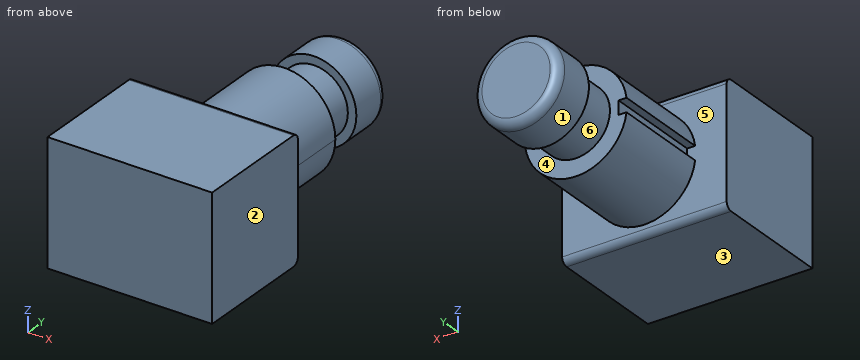
Autodesk Inventor part; units mm, degrees
ref_plane "YZ Plane" through (0, 0, 0) normal (1, 0, 0) x (0, 1, 0)
ref_plane "XZ Plane" through (0, 0, 0) normal (0, 1, 0) x (-1, 0, 0)
ref_plane "XY Plane" through (0, 0, 0) normal (0, 0, 1) x (1, 0, 0)
sketch "Sketch1" plane through (0, 0, 0) normal (0, 1, 0) x (-1, 0, 0)
  line L0 (9.65, 7.25) -> (-9.65, 7.25)
  line L1 (-9.65, 7.25) -> (-9.65, -7.25)
  line L2 (-9.65, -7.25) -> (9.65, -7.25)
  line L3 (9.65, -7.25) -> (9.65, 7.25)
  line L4 (9.65, 7.25) -> (-9.65, -7.25) construction
  line L5 (-9.65, 7.25) -> (9.65, -7.25) construction
  point P0 (0, 0)
  dimension "d0" = 19.3
  dimension "d1" = 14.5
extrude "Extrusion1" add sketch "Sketch1" along normal blind 14.5
sketch "Sketch2" plane through (0, 14.5, 0) normal (0, 1, 0) x (1, 0, 0)
  circle A0 centre (0, 0) radius 6
  line L0 (-6.9823, -0.8) -> (-5.0177, -0.8)
  line L1 (-5.0177, -0.8) -> (-5.0177, 0.8)
  line L2 (-5.0177, 0.8) -> (-6.9823, 0.8)
  line L3 (-6.9823, 0.8) -> (-6.9823, -0.8)
  line L4 (-6.9823, -0.8) -> (-5.0177, 0.8) construction
  line L5 (-5.0177, -0.8) -> (-6.9823, 0.8) construction
  point P0 (-6, 0)
  point P1 (5.9823, -0.4609)
  point P2 (-5.9464, -0.8)
  point P3 (-5.9464, 0.8)
  dimension "d4" = 12
  dimension "d5" = 1.6
  dimension "d6" = 11
extrude "Extrusion2" add sketch "Sketch2" along normal blind 11.6 contours A0 L0 L1 L2 picked at (-1.3451, 0)
sketch "Sketch3" plane through (0, 26.1, 0) normal (0, 1, 0) x (1, 0, 0)
  circle A0 centre (0, 0) radius 4
  dimension "d9" = 8
extrude "Extrusion3" add sketch "Sketch3" along normal blind 5
sketch "Sketch4" plane through (0, 31.1, 0) normal (0, 1, 0) x (1, 0, 0)
  circle A0 centre (0, 0) radius 5
  dimension "d12" = 10
extrude "Extrusion4" add sketch "Sketch4" along normal blind 5.1
fillet "Fillet1" radius 1 1 edges at (-5, 36.2, 0)
thread "Thread1"
fillet "Fillet2" radius 0.75 2 edges at (0, 14.5, 7.25) (0, 14.5, -7.25)
properties part number "ar70736"
The listing builds one solid part. Answer for the finished solid, in the listing's coordinates (mm). Face numbers are marked on the shaded views. A direction names the side the tool comes from. Coordinates: 2 decimals unless noted, no trailing zeros. Loops run counter-clockwise (first coordinate to the right, second up) from the corner with the lowest first, then second, coordinate; pieces in that order, holes last. Notation, with made-up numbers: (76, 80) -> (122, 80) arc R20 ccw to (122, 112) -> close; hole circle Ø9 at (58.5, 14.5). An arc over 180 degrees is marked (long way). Use one line per item in the form item = value. Start each with the question number.
Item 1: The part is cut by section C-C on y = 19.5. Determine the outline of the cut face in (x, z).
Item 2: The part is cut by section D-D on x = 0. Determine the outline of the cut face in (y, z).
Item 3: A tool of negligible diameter and unlimited length cuts with its end or side. For the marked faces 1 and 2, from which of +Z, -Z, +X, -X, +Y, -Y can it reach the whole face along a straight path? Write none if from no direction.
Item 4: Flat-ended cylindrical pins translate along their axes: pin 1 Ø0.5 at (x, y) = (-5.5, 18) entering from -Z; pin 2 Ø3 at (x, y) = (0.5, 29) entering from +Z; pin 3 Ø3 at (x, z) = (-6.5, 2) entering from +Y. Find the tip coordinate at first contact, or state that the pin passes through.
Item 5: The mould has two halves that part along Y. Classify the marked faces 3, 4, 5 and 6: released by +Y, released by -Y, zero draft, split by the parting line, or undercut.
Item 6: Consider L1, parallel to Y at x = 5.5, z = 6.25; L2, parallel to Y at x = 3.5, z = -4; L3, parallel to Z at x = 4, y = 24. Determine where each line is inside the solid, lowest interval first. Write a range as [from, to].
Item 7: The part is cut by section A-A on x = 7.5. Determine the outline of the cut face in (y, z), then the cut area to 3 significant figures.
Item 8: The part is cut by section B-B on z = 5.5. Determine the outline of the cut face in (x, y), then the cut area to 3 significant figures.
Answer key:
q1.outline = (-5.95, -0.8) arc R6 ccw (long way) to (-5.95, 0.8) -> (-5.02, 0.8) -> (-5.02, -0.8) -> close
q2.outline = (0, -7.25) -> (13.75, -7.25) arc R0.75 ccw to (14.5, -6.5) -> (14.5, -6) -> (26.1, -6) -> (26.1, -4) -> (31.1, -4) -> (31.1, -5) -> (35.2, -5) arc R1 ccw to (36.2, -4) -> (36.2, 4) arc R1 ccw to (35.2, 5) -> (31.1, 5) -> (31.1, 4) -> (26.1, 4) -> (26.1, 6) -> (14.5, 6) -> (14.5, 6.5) arc R0.75 ccw to (13.75, 7.25) -> (0, 7.25) -> close
q3.face_1 = +Y
q3.face_2 = +Z, -Z, +X, +Y, -Y
q4.pin_1 = -2.9
q4.pin_2 = 4
q4.pin_3 = 26.1
q5.face_3 = zero draft
q5.face_4 = undercut
q5.face_5 = released by +Y
q5.face_6 = undercut
q6.L1 = [0, 14.5]
q6.L2 = [0, 26.1]
q6.L3 = [-4.47, 4.47]
q7.outline = (0, -7.25) -> (13.75, -7.25) arc R0.75 ccw to (14.5, -6.5) -> (14.5, 6.5) arc R0.75 ccw to (13.75, 7.25) -> (0, 7.25) -> close
q7.area = 210 mm2
q8.outline = (-9.65, 0) -> (9.65, 0) -> (9.65, 14.5) -> (2.4, 14.5) -> (2.4, 26.1) -> (-2.4, 26.1) -> (-2.4, 14.5) -> (-9.65, 14.5) -> close
q8.area = 335 mm2
